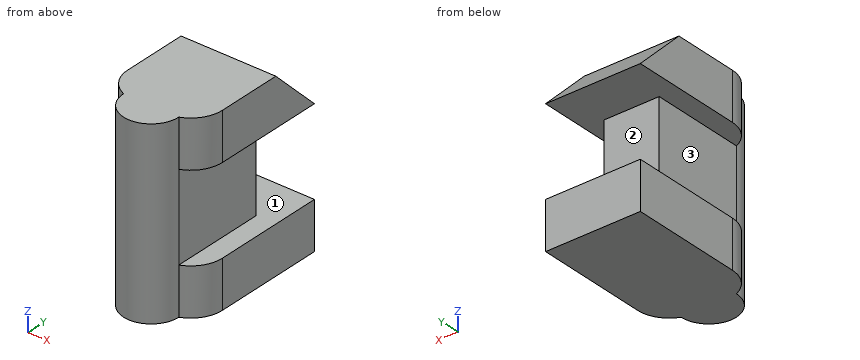
from build123d import *

# Parameters (mm, degrees)
F0_W        = 3.5
F0_H        = 5.5
F1_DEPTH    = 6
F2_W        = 1.75
F2_H        = 11.5
F4_T1_DEPTH = 12.2702481089
F4_T3_DEPTH = 12.2702481089
F5_W        = 6
F5_H        = 3
F6_DEPTH    = 3
F8_DEPTH    = 25


# Not quite as in the source:
# - a fillet or chamfer that OpenCascade refuses, or shapes differently, is made with other operations: its cross-section is extruded or revolved along the edge and cut away or added


with BuildPart() as f1:
    # F0 (on Front) → F1 (new body)
    with BuildSketch(Plane.XZ):
        Polygon((1.75, -1.5), (3, -1.5), (3, 1.5), (-3, 1.5), (-3, -1.5), (-1.75, -1.5), align=None)
        with Locations((0, -4.25)):
            Rectangle(F0_W, F0_H)
        Polygon((3, -7), (1.75, -7), (-1.75, -7), (-3, -7), (-3, -10), (3, -10), align=None)
    extrude(amount=F1_DEPTH)

    # F2 (on face) → F3 (revolve)
    with BuildSketch(Plane.XZ.offset(6)):
        with Locations((-0.875, -4.25)):
            Rectangle(F2_W, F2_H)
    revolve(axis=Axis((0, -6, -4.25), (0, 0, -1)))

    # F4: fillet of radius 2 on 4 edges, made by hand

    # F4_s2 → F4_t1 (cut)
    with BuildSketch(Plane.XY.offset(-6.1351240544)):
        with BuildLine():
            ThreePointArc((3, -4.1459503782), (2.6583123952, -5.263984367), (1.75, -6))
            Line((1.75, -6), (3, -6))
            Line((3, -6), (3, -4.1459503782))
        make_face()
        with BuildLine():
            ThreePointArc((-3, -4.1459503782), (-2.6583123952, -5.263984367), (-1.75, -6))
            Line((-1.75, -6), (-3, -6))
            Line((-3, -6), (-3, -4.1459503782))
        make_face()
    extrude(amount=F4_T1_DEPTH, mode=Mode.SUBTRACT)

    # F4_s4 → F4_t3 (cut)
    with BuildSketch(Plane.XY.offset(-14.6351240544)):
        with BuildLine():
            ThreePointArc((3, -4.1459503782), (2.6583123952, -5.263984367), (1.75, -6))
            Line((1.75, -6), (3, -6))
            Line((3, -6), (3, -4.1459503782))
        make_face()
        with BuildLine():
            ThreePointArc((-3, -4.1459503782), (-2.6583123952, -5.263984367), (-1.75, -6))
            Line((-1.75, -6), (-3, -6))
            Line((-3, -6), (-3, -4.1459503782))
        make_face()
    extrude(amount=F4_T3_DEPTH, mode=Mode.SUBTRACT)

    # F5 (on face) → F6 (join)
    with BuildSketch(Plane(origin=(0, 0, 0), x_dir=(-1, 0, 0), z_dir=(0, 1, 0))):
        Rectangle(F5_W, F5_H)
        with Locations((0, -8.5)):
            Rectangle(F5_W, F5_H)
    extrude(amount=F6_DEPTH)

    # F7 (on face) → F8 (cut)
    with BuildSketch(Plane.YZ.offset(3)):
        Polygon((0, 1.5), (3, -1.5), (3, 1.5), align=None)
    extrude(amount=-F8_DEPTH, mode=Mode.SUBTRACT)


solid = f1.part
Design review of the part built by this model. Coordinates are the model's own, in mm. Face numbers are marked on the shaded views. A direction names the side the tool comes from. Coordinates: 2 decimals unless noted, no trailing zeros. Loops run counter-clockwise (first coordinate to the right, second up) from the corner with the lowest first, then second, coordinate; pieces in that order, holes last. Notation, with made-up numbers: M 77,84.5 L 92,84.5 A23 cw 92,115.5 Z; hole C 49.25,26.5 d11. An arc over 180 degrees is marked long. Answer as CSV lines item,"result".
Item 1: For probe 1 along Z at (x, y) = (2, -4.5); probe 2 along X at (y, z) = (-0.5, -4.75); probe 3 along Z at (x, y) = (-0.5, 1), list the stretches that pass through material, from the lowest coordinate up.
Answer list:
probe 1,"-10 to -7, -1.5 to 1.5"
probe 2,"-1.75 to 1.75"
probe 3,"-10 to -7, -1.5 to 0.5"
Item 2: Add section A-A on y = 1. State the section outline as (x, z) points, plus the area to 3 significant figures.
Answer list:
outline,"M -3,-10 L 3,-10 L 3,-7 L -3,-7 Z; M -3,-1.5 L 3,-1.5 L 3,0.5 L -3,0.5 Z"
area,"30.0 mm²"
Item 3: Machinability: for the marked faces 1, 2 and 3, which of the approach directions +Z, -Z, +X, -X, +Y, -Y give a long, thin tool a straight path to every point of the face, cutting with its end or side? Answer none if there is none.
Answer list:
face 1,"+Y"
face 2,"+X, -X, +Y"
face 3,"-X, +Y, -Y"
Item 4: Add section B-B on x = 2. State the section outline as (y, z) points, plus the area to 3 significant figures.
Answer list:
outline,"M -5.88,-10 L 3,-10 L 3,-7 L -5.88,-7 Z; M -5.88,-1.5 L 3,-1.5 L 0,1.5 L -5.88,1.5 Z"
area,"48.8 mm²"
Item 5: For P1, Ø6, axis at y = -5, z = -7, coming from the +X side, flat-tipped, find the tip position at first contact; note if it passes through.
Answer list:
P1,"x = 3"
Item 6: Add section D-D on y = -3.75. State the section outline as (x, z) points, plus the area to 4 significant figures.
Answer list:
outline,"M -3,-10 L 3,-10 L 3,-7 L 1.75,-7 L 1.75,-1.5 L 3,-1.5 L 3,1.5 L -3,1.5 L -3,-1.5 L -1.75,-1.5 L -1.75,-7 L -3,-7 Z"
area,"55.25 mm²"
Item 7: Add section C-C on z = -1. State the section outline as (x, y) points, plus the area to 3 significant figures.
Answer list:
outline,"M -3,-4.15 A2 ccw -1.75,-6 A1.75 ccw 1.75,-6 A2 ccw 3,-4.15 L 3,2.5 L -3,2.5 Z"
area,"54.5 mm²"
